The model under review builds one solid part; all positions refer to its coordinate system, in mm. Coordinates: 2 decimals unless noted, no trailing zeros. Write each loop counter-clockwise with the first axis right and the second up, starting at its lowest first coordinate (ties: lowest second). Pieces come first, ordered by that corner, then holes. Notation, with made-up numbers: (-11.5, 16) - (23.5, 16) arc R9 cw to (23.5, 29) - close; hole circle Ø2 at (-10, 7). An arc over 180 degrees is marked (long way). Put each result on its own line as item: value. Start each with the question number.
Item 1: For pin 1 (4 mm diameter, centred on y = 26.1, z = -11.62, fed in from -X); pin 2 (2.5 mm diameter, centred on y = 8.83, z = 27.18, fed in from +X); pin 3 (1 mm diameter, centred on x = 0.5, y = 3.5, fed in from +Z); pin 4 (1.5 mm diameter, centred on x = 1, y = -2, fed in from +Z), all flat-tipped, find the tip position at first contact; note any pin that passes through.
Item 2: Consider section B-B on z = 0. Give the boundary of the cut face in (x, y) (3 decimals), then the cut area to 3 significant figures.
Item 3: To check wall thickness, follow L1, parallel to Y at x = 1, z = -1; L2, parallel to Y at x = 2.1, z = 0 (3 decimals); L3, parallel to Z at x = 1, y = 19.5. State the ranges of each line that lie inside material, in increasing order. Write a range as [from, to].
Item 4: Consider section D-D on y = 22. Give the boundary of the cut face in (x, z) (3 decimals), then the cut area to 3 significant figures.
Item 5: Consider section C-C on x = 2.6. State how many separate pieces and enclosed holes the cut face has, then the cut area to 3 significant figures.
Item 6: Consider section A-A on y = 0. Give the boundary of the cut face in (x, z) (3 decimals).
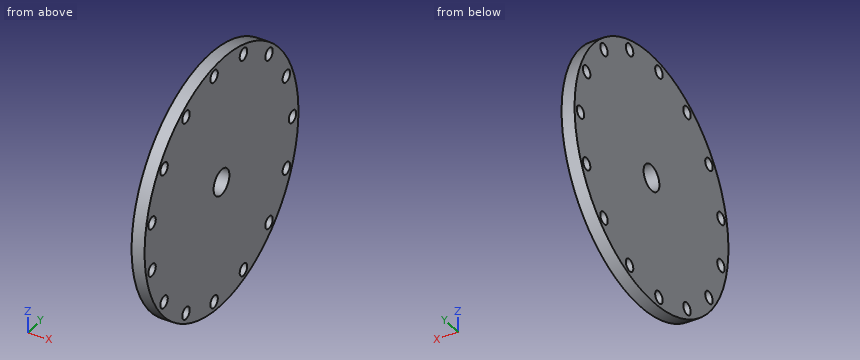
```python
from build123d import *

# Parameters (mm, degrees)
SKETCH1_R           = 30.95625
SKETCH1_R_2         = 1.5
BOSS_EXTRUDE1_DEPTH = 3.175
SKETCH2_R           = 3.175
CUT_EXTRUDE1_DEPTH  = 44.893729087


with BuildPart() as part:
    # Sketch1 → Boss-Extrude1 (new body)
    with BuildSketch(Plane(origin=(0, 0, 0), x_dir=(0, 0, -1), z_dir=(1, 0, 0))):
        Circle(SKETCH1_R)
        with Locations((0, 28.575)):
            Circle(SKETCH1_R_2, mode=Mode.SUBTRACT)
        with Locations((11.622499576, 26.104561452)):
            Circle(SKETCH1_R_2, mode=Mode.SUBTRACT)
        with Locations((21.235363388, 19.120407077)):
            Circle(SKETCH1_R_2, mode=Mode.SUBTRACT)
        with Locations((27.176439953, 8.830160614)):
            Circle(SKETCH1_R_2, mode=Mode.SUBTRACT)
        with Locations((28.41846316, -2.986900838)):
            Circle(SKETCH1_R_2, mode=Mode.SUBTRACT)
        with Locations((24.746675913, -14.2875)):
            Circle(SKETCH1_R_2, mode=Mode.SUBTRACT)
        with Locations((16.795963584, -23.117660614)):
            Circle(SKETCH1_R_2, mode=Mode.SUBTRACT)
        with Locations((5.941076565, -27.950567691)):
            Circle(SKETCH1_R_2, mode=Mode.SUBTRACT)
        with Locations((-5.941076565, -27.950567691)):
            Circle(SKETCH1_R_2, mode=Mode.SUBTRACT)
        with Locations((-16.795963584, -23.117660614)):
            Circle(SKETCH1_R_2, mode=Mode.SUBTRACT)
        with Locations((-24.746675913, -14.2875)):
            Circle(SKETCH1_R_2, mode=Mode.SUBTRACT)
        with Locations((-28.41846316, -2.986900838)):
            Circle(SKETCH1_R_2, mode=Mode.SUBTRACT)
        with Locations((-27.176439953, 8.830160614)):
            Circle(SKETCH1_R_2, mode=Mode.SUBTRACT)
        with Locations((-21.235363388, 19.120407077)):
            Circle(SKETCH1_R_2, mode=Mode.SUBTRACT)
        with Locations((-11.622499576, 26.104561452)):
            Circle(SKETCH1_R_2, mode=Mode.SUBTRACT)
    extrude(amount=BOSS_EXTRUDE1_DEPTH)

    # Sketch2 → Cut-Extrude1 (cut, through all)
    with BuildSketch(Plane(origin=(3.175, 0, 0), x_dir=(0, 0, -1), z_dir=(1, 0, 0))):
        Circle(SKETCH2_R)
    extrude(amount=-CUT_EXTRUDE1_DEPTH, mode=Mode.SUBTRACT)


solid = part.part
```
Report:
1. pin 1: x = 0
1. pin 2: through
1. pin 3: z = 30.81
1. pin 4: z = 30.93
2. outline: (0, -30.956) - (3.175, -30.956) - (3.175, -3.175) - (0, -3.175) - close; (0, 3.175) - (3.175, 3.175) - (3.175, 27.075) - (0, 27.075) - close; (0, 30.075) - (3.175, 30.075) - (3.175, 30.956) - (0, 30.956) - close
2. area: 167 mm²
3. L1: [-30.94, -3.01], [3.01, 27.46], [29.69, 30.94]
3. L2: [-30.956, -3.175], [3.175, 27.075], [30.075, 30.956]
3. L3: [-24.04, -22.69], [-19.78, 19.78], [22.69, 24.04]
4. outline: (0, -21.778) - (3.175, -21.778) - (3.175, 21.778) - (0, 21.778) - close
4. area: 138 mm²
5. separate pieces: 1
5. enclosed holes: 16
5. area: 2,870 mm²
6. outline: (0, -30.956) - (3.175, -30.956) - (3.175, -3.175) - (0, -3.175) - close; (0, 3.175) - (3.175, 3.175) - (3.175, 30.956) - (0, 30.956) - close
